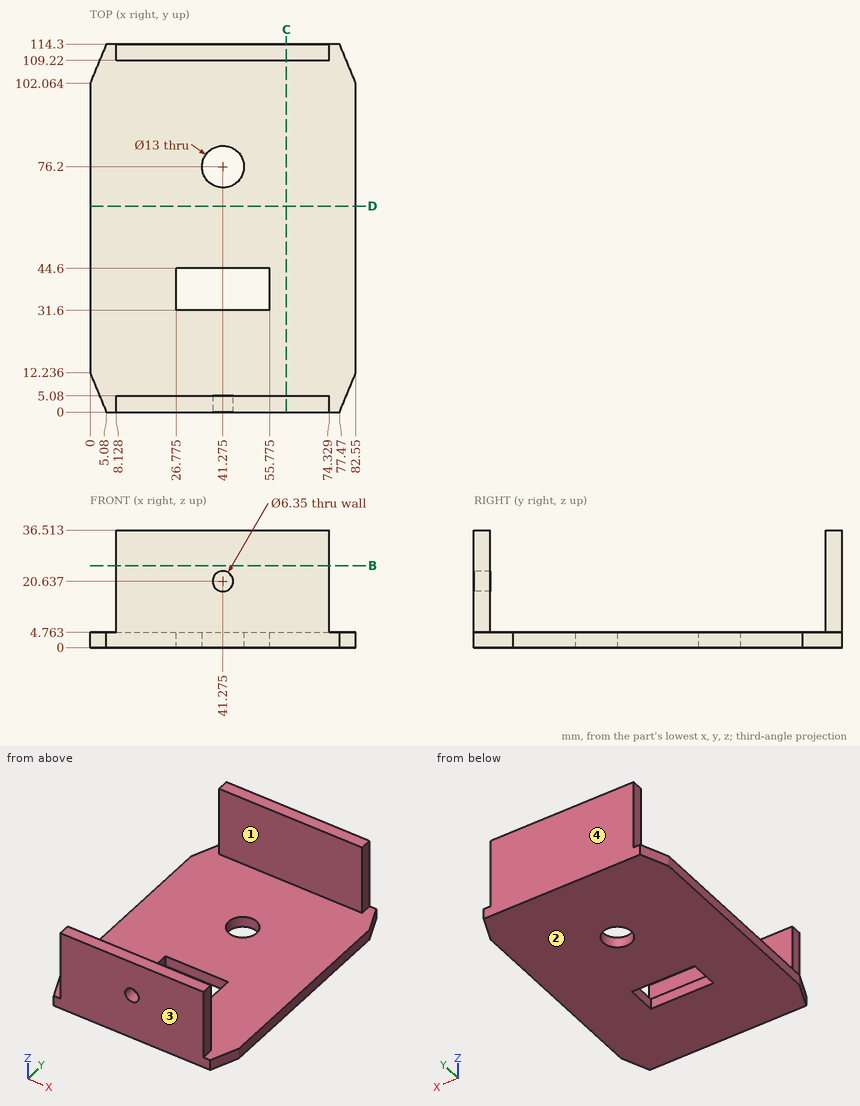
Here's the drawing with two shaded views (mm, measured from the low corner). I have some questions. Round coordinates to 2 decimals unless told otherwise and drop trailing zeros. Order: outer loops, then holes, each group sorted by start corner. A loop starts at its lowest first (then second) coordinate and runs counter-clockwise, first axis right, second up. Notation, with made-up numbers: M -11.75,3 L 13.25,3 A15 ccw 13.25,14 Z; hole C 62.5,45.5 d4. An arc over 180 degrees is marked long. Answer in a Markdown table with one row per item.
Item 1: Imagine slicing it at D-D, the plane y = 64. Write out the boundary of the cut face in (x, z).
A:
| item | result |
|---|---|
| outline | M 0,0 L 82.55,0 L 82.55,4.76 L 0,4.76 Z |
Item 2: Thinking about a two-plate mould opening in Y: for the marked faces 1, 2, 3 and 4, which applies, +Y half, -Y half, draft (parallel to the pull), parting line (faces both ways), or undercut?
A:
| item | result |
|---|---|
| face 1 | undercut |
| face 2 | draft |
| face 3 | -Y half |
| face 4 | +Y half |
Item 3: Imagine slicing it at B-B, the plane z = 25.5. Write out the boundary of the cut face in (x, y).
A:
| item | result |
|---|---|
| outline | M 8.13,0 L 74.33,0 L 74.33,5.08 L 8.13,5.08 Z; M 8.13,109.22 L 74.33,109.22 L 74.33,114.3 L 8.13,114.3 Z |
Item 4: I'm going to push flat-ended pins straight in: pin 1 (5 mm diameter, centred on x = 35, z = 14, fed in from -Y); pin 2 (2.5 mm diameter, centred on y = 110.5, z = 14, fed in from -X); pin 3 (5 mm diameter, centred on x = 74, y = 40.5, fed in from +Z); pin 4 (4 mm diameter, centred on y = 112, z = 17, fed in from +X). Where does each tip first touch, or does it pass through?
A:
| item | result |
|---|---|
| pin 1 | stops at y = 0 |
| pin 2 | stops at x = 8.13 |
| pin 3 | stops at z = 4.76 |
| pin 4 | stops at x = 74.33 |
Item 5: If I drill on L1, parallel to Y at x = 18, z = 27.5; L2, parallel to Y at x = 49, z = 4.5; L3, parallel to X at y = 76, z = 3, over which ranges is the centre line in solid material (lowest first)? Write a range as from..to.
A:
| item | result |
|---|---|
| L1 | y = 0..5.08, 109.22..114.3 |
| L2 | y = 0..31.6, 44.6..114.3 |
| L3 | x = 0..34.78, 47.77..82.55 |
Item 6: Imagine slicing it at C-C, the plane x = 61. Write out the boundary of the cut face in (y, z), and give its area (3 significant figures).
A:
| item | result |
|---|---|
| outline | M 0,0 L 114.3,0 L 114.3,36.51 L 109.22,36.51 L 109.22,4.76 L 5.08,4.76 L 5.08,36.51 L 0,36.51 Z |
| area | 867 mm2 |
